Read the model definition and answer for the solid it produces. Units are mm, in the model's axes. Coordinates: 2 decimals unless noted, no trailing zeros. Order: outer loops, then holes, each group sorted by start corner. A loop starts at its lowest first (then second) coordinate and runs counter-clockwise, first axis right, second up.
```python
from build123d import *

# Parameters (mm, degrees)
SKETCH1_R           = 4
BOSS_EXTRUDE1_DEPTH = 3.175
SKETCH2_R           = 4
SKETCH2_R_2         = 2.95
BOSS_EXTRUDE2_DEPTH = 3.175


with BuildPart() as part:
    # Sketch1 → Boss-Extrude1 (new body)
    with BuildSketch(Plane(origin=(0, 0, 0), x_dir=(1, 0, 0), z_dir=(0, 1, 0))):
        with BuildLine():
            ThreePointArc((1.961570561, 9.861481147), (0, 12.251661791), (-1.961570561, 9.861481147))
            ThreePointArc((-1.961570561, 9.861481147), (-3.157774257, 7.623541438), (-5.586080346, 8.360160037))
            ThreePointArc((-5.586080346, 8.360160037), (-8.663233133, 8.663233133), (-8.360160037, 5.586080346))
            ThreePointArc((-8.360160037, 5.586080346), (-7.623541438, 3.157774257), (-9.861481147, 1.961570561))
            ThreePointArc((-9.861481147, 1.961570561), (-12.251661791, 0), (-9.861481147, -1.961570561))
            ThreePointArc((-9.861481147, -1.961570561), (-7.623541438, -3.157774257), (-8.360160037, -5.586080346))
            ThreePointArc((-8.360160037, -5.586080346), (-8.663233133, -8.663233133), (-5.586080346, -8.360160037))
            ThreePointArc((-5.586080346, -8.360160037), (-3.157774257, -7.623541438), (-1.961570561, -9.861481147))
            ThreePointArc((-1.961570561, -9.861481147), (0, -12.251661791), (1.961570561, -9.861481147))
            ThreePointArc((1.961570561, -9.861481147), (3.157774257, -7.623541438), (5.586080346, -8.360160037))
            ThreePointArc((5.586080346, -8.360160037), (8.663233133, -8.663233133), (8.360160037, -5.586080346))
            ThreePointArc((8.360160037, -5.586080346), (7.623541438, -3.157774257), (9.861481147, -1.961570561))
            ThreePointArc((9.861481147, -1.961570561), (12.251661791, 0), (9.861481147, 1.961570561))
            ThreePointArc((9.861481147, 1.961570561), (7.623541438, 3.157774257), (8.360160037, 5.586080346))
            ThreePointArc((8.360160037, 5.586080346), (8.663233133, 8.663233133), (5.586080346, 8.360160037))
            ThreePointArc((5.586080346, 8.360160037), (3.157774257, 7.623541438), (1.961570561, 9.861481147))
        make_face()
        Circle(SKETCH1_R, mode=Mode.SUBTRACT)
    extrude(amount=BOSS_EXTRUDE1_DEPTH)

    # Sketch2 → Boss-Extrude2 (add)
    with BuildSketch(Plane(origin=(0, 3.175, 0), x_dir=(1, 0, 0), z_dir=(0, 1, 0))):
        Circle(SKETCH2_R)
        Circle(SKETCH2_R_2, mode=Mode.SUBTRACT)
    extrude(amount=-BOSS_EXTRUDE2_DEPTH)


solid = part.part
```
1) A cutting plane is placed at A-A, the plane z = 0. Determine the outline of the cut face in (x, y) (3 decimals).
A:
outline: (-12.252, 0) - (-2.95, 0) - (-2.95, 3.175) - (-12.252, 3.175) - close; (2.95, 0) - (12.252, 0) - (12.252, 3.175) - (2.95, 3.175) - close
2) Straight lines are drawn through the part: line 1 (X direction, y = 3, z = -8.75); line 2 (X direction, y = 0.15, z = -8); line 3 (X direction, y = 2.1, z = 1.75). For each, find the intervals that lie inside material, in ascending order.
A:
line 1: x = -8.57 to -5.93, -2.06 to 2.06, 5.93 to 8.57
line 2: x = -9.1 to -5.28, -2.57 to 2.57, 5.28 to 9.1
line 3: x = -11.22 to -2.37, 2.37 to 11.22
3) A cutting plane is placed at C-C, the plane z = 7.75. Determine the outline of the cut face in (x, y) (3 decimals), and give its area (3 significant figures).
A:
outline: (-9.185, 0) - (-4.942, 0) - (-4.942, 3.175) - (-9.185, 3.175) - close; (-2.905, 0) - (2.905, 0) - (2.905, 3.175) - (-2.905, 3.175) - close; (4.942, 0) - (9.185, 0) - (9.185, 3.175) - (4.942, 3.175) - close
area: 45.4 mm2
4) Flat-ended cylindrical pins translate along their axes: pin 1 Ø5.5 at (x, z) = (0, 0) entering from -Y; pin 2 Ø1.5 at (y, z) = (2, 1) entering from -X; pin 3 Ø4 at (x, z) = (-8, 1.5) entering from -Y; pin 4 Ø1.5 at (y, z) = (2.5, 3) entering from -X. Find the tip coordinate at first contact, or state that the pin passes through.
A:
pin 1: passes through
pin 2: stops at x = -12.24
pin 3: stops at y = 0
pin 4: stops at x = -8.38
5) A cutting plane is placed at D-D, the plane y = 2.75. Determine the outline of the cut face in (x, z), and give its area (3 significant figures).
A:
outline: (-9.86, -1.96) arc R2 cw to (-8.36, -5.59) arc R2 ccw (long way) to (-5.59, -8.36) arc R2 cw to (-1.96, -9.86) arc R2 ccw (long way) to (1.96, -9.86) arc R2 cw to (5.59, -8.36) arc R2 ccw (long way) to (8.36, -5.59) arc R2 cw to (9.86, -1.96) arc R2 ccw (long way) to (9.86, 1.96) arc R2 cw to (8.36, 5.59) arc R2 ccw (long way) to (5.59, 8.36) arc R2 cw to (1.96, 9.86) arc R2 ccw (long way) to (-1.96, 9.86) arc R2 cw to (-5.59, 8.36) arc R2 ccw (long way) to (-8.36, 5.59) arc R2 cw to (-9.86, 1.96) arc R2 ccw (long way) to start; hole circle Ø5.9 at (0, 0)
area: 307 mm2
6) Determine the mould class of faces 1 (the flat face through (-3, 0, -3)), 2 (the cylindrical face through (-2.947, 1.61, -0.13)) for opening direction X: pulls with the +X half, pulls with the -X half, needs draft (parallel to the pull), parting line crosses it, or undercut.
A:
face 1: needs draft
face 2: undercut
7) A cutting plane is placed at B-B, the plane x = 0. Determine the outline of the cut face in (y, z) (3 decimals).
A:
outline: (0, -12.252) - (3.175, -12.252) - (3.175, -2.95) - (0, -2.95) - close; (0, 2.95) - (3.175, 2.95) - (3.175, 12.252) - (0, 12.252) - close
